Check sheet for the drawn part. Datum: minimum x, y, z corner. Units: mm. Coordinates: 2 decimals unless noted, no trailing zeros. Loops run counter-clockwise (first coordinate to the right, second up) from the corner with the lowest first, then second, coordinate; pieces in that order, holes last.
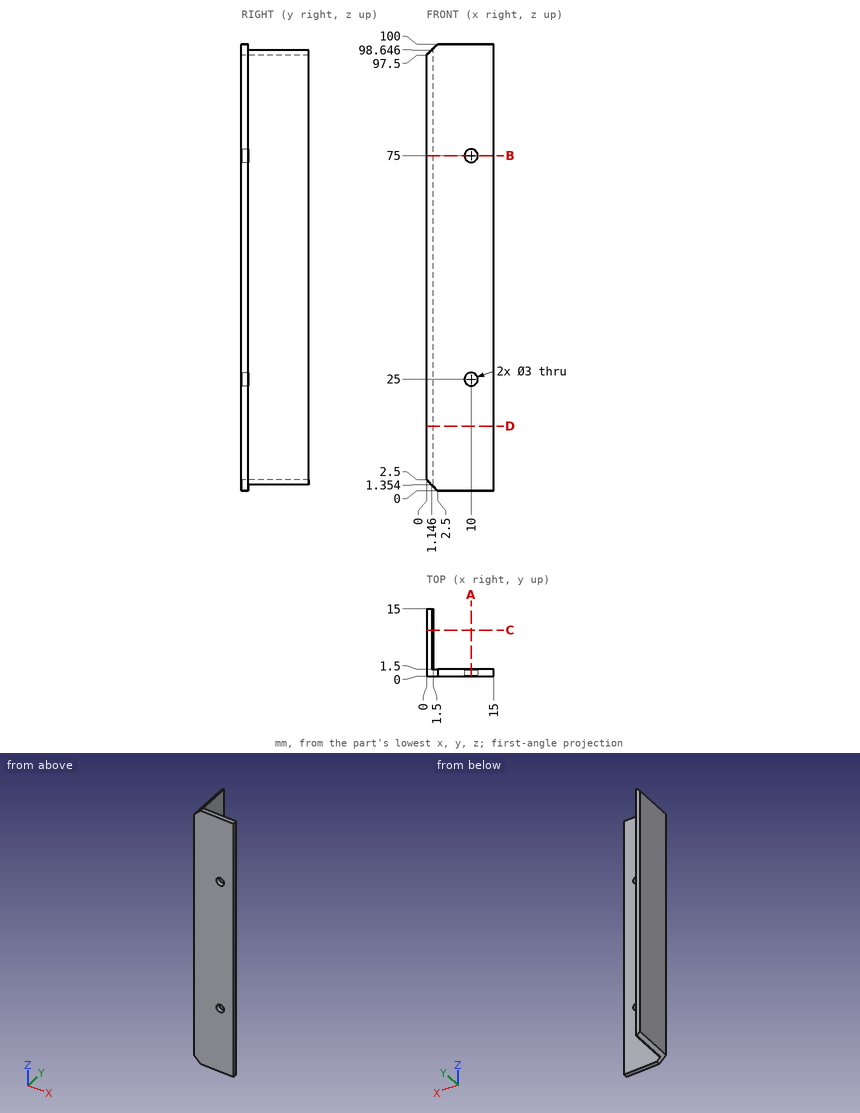
(1) Sectioned sample at C-C on y = 10.25. Record the cut outline in (x, z).
Findings:
outline: (0, 2.5) - (1.15, 1.35) - (1.5, 1.35) - (1.5, 98.65) - (1.15, 98.65) - (0, 97.5) - close
(2) Gauge pin test, flat ends, axial feed: pin 1 Ø7 at (y, z) = (7.5, 51.5) entering from +X; pin 2 Ø1.5 at (x, z) = (8.5, 30.5) entering from +Y. Record the tip position at first contact, or that the pin passes through.
Findings:
pin 1: stops at x = 1.5
pin 2: stops at y = 1.5
(3) Sectioned sample at D-D on z = 14.5. Record the cut outline in (x, y).
Findings:
outline: (0, 0) - (15, 0) - (15, 1.5) - (1.5, 1.5) - (1.5, 15) - (0, 15) - close
(4) Sectioned sample at B-B on z = 75. Record the cut outline in (x, y).
Findings:
outline: (0, 0) - (8.5, 0) - (8.5, 1.5) - (1.5, 1.5) - (1.5, 15) - (0, 15) - close; (11.5, 0) - (15, 0) - (15, 1.5) - (11.5, 1.5) - close
(5) Scan lines: L1, parallel to X at y = 1, z = 25; L2, parallel to Y at x = 6, z = 73. Record each from-to range of solid material in increasing order.
Findings:
L1: x = 0 to 8.5, 11.5 to 15
L2: y = 0 to 1.5
(6) Sectioned sample at A-A on x = 10. Record the cut outline in (y, z).
Findings:
outline: (0, 0) - (1.5, 0) - (1.5, 23.5) - (0, 23.5) - close; (0, 26.5) - (1.5, 26.5) - (1.5, 73.5) - (0, 73.5) - close; (0, 76.5) - (1.5, 76.5) - (1.5, 100) - (0, 100) - close
